Can you work these out from the model? Positions are in its coordinate system, mm. Face numbers are marked on the shaded views. A direction names the side the tool comes from. Give positions to 0.01 mm unless a question says otherwise; leave off trailing zeros. Order: outer loops, then holes, each group sorted by start corner. A loop starts at its lowest first (then second) coordinate and runs counter-clockwise, first axis right, second up. Notation, with made-up numbers: M -31.75,29 L 8.25,29 A10 ccw 8.25,45 Z; hole C 40.5,-22.75 d10. An arc over 180 degrees is marked long. Use a Markdown table: item, result. Add a question column.
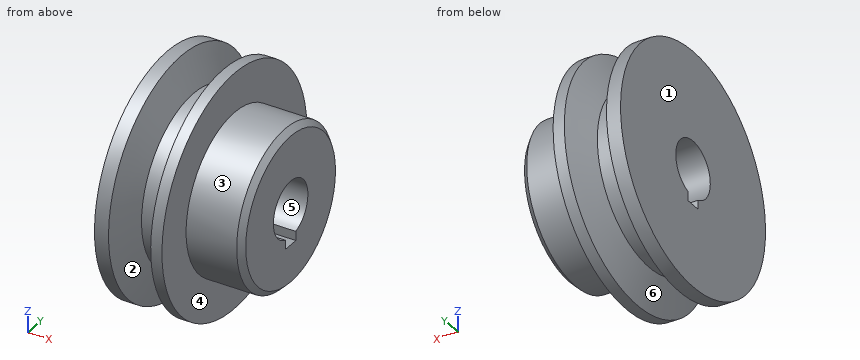
from build123d import *

# Parameters (mm, degrees)
CHAMFER1_SIZE      = 1
CUT_EXTRUDE1_REACH = 38.959


with BuildPart() as part:
    # Sketch1 → Revolve1 (revolve)
    with BuildSketch(Plane.XY, mode=Mode.PRIVATE) as revolve1_sk:
        Polygon((-12, 5), (10, 5), (10, 14), (0, 14), (0, 21), (-2, 21), (-4.183821406, 15), (-7.316178594, 15), (-9.5, 21), (-12, 21), align=None)
    revolve(revolve1_sk.sketch.rotate(Axis((-92.477937902, 0, 0), (1, 0, 0)), 90), axis=Axis((-92.477937902, 0, 0), (1, 0, 0)))

    # Chamfer1
    chamfer1_edges = [part.edges().sort_by_distance(p)[0] for p in [
        (10, 0, -14),
    ]]
    chamfer(chamfer1_edges, length=CHAMFER1_SIZE)

    # Sketch2 → Cut-Extrude1 (cut, up to next)
    with BuildSketch(Plane(origin=(10, 0, 0), x_dir=(0, 0, -1), z_dir=(1, 0, 0)), mode=Mode.PRIVATE) as cut_extrude1_sk1:
        with BuildLine():
            Line((4.769696007, 1.5), (6.4, 1.5))
            Line((6.4, 1.5), (6.4, -1.5))
            Line((6.4, -1.5), (4.769696007, -1.5))
            ThreePointArc((4.769696007, -1.5), (5, 0), (4.769696007, 1.5))
        make_face()
    cut_extrude1_tool1 = extrude(cut_extrude1_sk1.sketch, amount=-CUT_EXTRUDE1_REACH, mode=Mode.PRIVATE) & part.part
    add(cut_extrude1_tool1.solids().sort_by_distance((10, 0, -5.660391))[0], mode=Mode.SUBTRACT)


solid = part.part
1. We'd pull the mould along X, two halves only. Please class the marked faces 1, 2 and 3: +X half, -X half, draft (parallel to the pull), parting line (faces both ways), or undercut.
2. Will these pins go through, and if not, where does the flat tip stop? pin 1 (0.9 mm diameter, centred on x = 4.5, y = 0, fed in from +Z); pin 2 (10 mm diameter, centred on x = -3, z = -8, fed in from -Y); pin 3 (1.5 mm diameter, centred on y = 13, z = -1.5, fed in from +X); pin 4 (10 mm diameter, centred on x = -9.5, z = -14.5, fed in from +Y).
3. On a 3-axis mill with a long thin cutter (end or side, diameter ignored), from which of +Z, -Z, +X, -X, +Y, -Y can I reach the whole of each face in a straight line? I mean the marked faces 4, 5 and 6. Say none if no direction works.
4. If we section it at A-A, the plane y = 0: List the corners of the cut face in (x, z) for me.
5. If we section it at D-D, the plane x = -5.75: List the corners of the cut face in (y, z) for me.
6. I need wall thicknesses on L1, parallel to Y at x = 1.25, z = 0; L2, parallel to Y at x = -4.75, z = 0; L3, parallel to X at y = -4, z = -15.5. Which ranges of each line are inside material? Lowest first, please. Write a range as [from, to].
7. If we section it at B-B, the plane z = 0: List the corners of the cut face in (x, y) for me.
8. If we section it at C-C, the plane x = 3.5: List the corners of the cut face in (y, z) for me.
Geometry results:
| question | item | result |
|---|---|---|
| 1 | face 1 | -X half |
| 1 | face 2 | undercut |
| 1 | face 3 | draft |
| 2 | pin 1 | stops at z = 14 |
| 2 | pin 2 | stops at y = -20.77 |
| 2 | pin 3 | stops at x = 10 |
| 2 | pin 4 | stops at y = 18.73 |
| 3 | face 4 | +X |
| 3 | face 5 | +X, -X |
| 3 | face 6 | none |
| 4 | outline | M -12,-21 L -9.5,-21 L -7.32,-15 L -4.18,-15 L -2,-21 L 0,-21 L 0,-14 L 9,-14 L 10,-13 L 10,-6.4 L -12,-6.4 Z; M -12,5 L 10,5 L 10,13 L 9,14 L 0,14 L 0,21 L -2,21 L -4.18,15 L -7.32,15 L -9.5,21 L -12,21 Z |
| 5 | outline | C 0,0 d30; hole M -1.5,-6.4 L 1.5,-6.4 L 1.5,-4.77 A5 ccw long -1.5,-4.77 Z |
| 6 | L1 | y = [-14, -5], [5, 14] |
| 6 | L2 | y = [-15, -5], [5, 15] |
| 6 | L3 | x = [-12, -7.68], [-3.82, 0] |
| 7 | outline | M -12,-21 L -9.5,-21 L -7.32,-15 L -4.18,-15 L -2,-21 L 0,-21 L 0,-14 L 9,-14 L 10,-13 L 10,-5 L -12,-5 Z; M -12,5 L 10,5 L 10,13 L 9,14 L 0,14 L 0,21 L -2,21 L -4.18,15 L -7.32,15 L -9.5,21 L -12,21 Z |
| 8 | outline | C 0,0 d28; hole M -1.5,-6.4 L 1.5,-6.4 L 1.5,-4.77 A5 ccw long -1.5,-4.77 Z |
